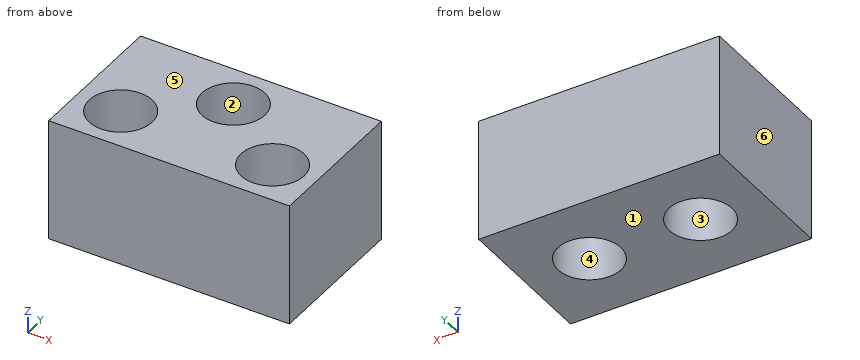
Autodesk Inventor part; units mm, degrees
ref_plane "YZ Plane" through (0, 0, 0) normal (1, 0, 0) x (0, 1, 0)
ref_plane "XZ Plane" through (0, 0, 0) normal (0, 1, 0) x (-1, 0, 0)
ref_plane "XY Plane" through (0, 0, 0) normal (0, 0, 1) x (1, 0, 0)
sketch "Sketch1" plane through (0, 0, 0) normal (0, 0, 1) x (1, 0, 0)
  line L0 (-30.2326, 17.8682) -> (11.0424, 17.8682)
  line L1 (11.0424, 17.8682) -> (11.0424, -7.5318)
  line L2 (11.0424, -7.5318) -> (-30.2326, -7.5318)
  line L3 (-30.2326, -7.5318) -> (-30.2326, 17.8682)
  point P0 (0, 0)
  dimension "d0" = 41.275
  dimension "d1" = 25.4
extrude "Extrusion1" add sketch "Sketch1" along normal blind 20.955
sketch "Sketch2" plane through (0, 0, 20.955) normal (0, 0, 1) x (1, 0, 0)
  line L0 (11.0424, 17.8682) -> (11.0424, -7.5318)
  line L1 (-30.2326, 17.8682) -> (11.0424, 17.8682)
  line L2 (-30.2326, -7.5318) -> (-30.2326, 17.8682)
  line L3 (11.0424, -7.5318) -> (-30.2326, -7.5318)
  circle A0 centre (-9.5951, 10.2482) radius 5.3975
  circle A1 centre (-22.6126, 0.0882) radius 5.3975
  circle A2 centre (3.4224, 0.0882) radius 5.3975
  dimension "d4" = 10.795
  dimension "d5" = 7.62
  dimension "d6" = 7.62
  dimension "d7" = 7.62
  dimension "d8" = 7.62
  dimension "d9" = 7.62
extrude "Extrusion2" cut sketch "Sketch2" against normal blind 9.525 contours A0 | A1 | A2
thread "Thread1"
thread "Thread2"
thread "Thread3"
sketch "Sketch3" plane through (0, 0, 0) normal (0, 0, -1) x (-1, 0, 0)
  line L0 (30.2326, -7.5318) -> (30.2326, 17.8682)
  circle A0 centre (0.0701, 5.1682) radius 5.3975
  circle A1 centre (19.1201, 5.1682) radius 5.3975
  point P0 (0, 0)
  dimension "d18" = 10.795
  dimension "d19" = 19.05
  dimension "d20" = 11.1125
extrude "Extrusion3" cut sketch "Sketch3" against normal blind 9.525
thread "Thread4"
thread "Thread5"
properties part number "Solenoid Base 1764"
Geometry check sheet. Reference: the model listing, model coordinates, mm. Face numbers are marked on the shaded views. A direction names the side the tool comes from. Round coordinates to 2 decimals unless told otherwise and drop trailing zeros. Loops run counter-clockwise (first coordinate to the right, second up) from the corner with the lowest first, then second, coordinate; pieces in that order, holes last. Notation, with made-up numbers: M 52,20.25 L 66,20.25 A27 ccw 66,53.25 Z; hole C -10.75,12 d7. An arc over 180 degrees is marked long. Return JSON: item names as keys, results as strings. Group by question number.
(1) Set-up check for the marked faces 1, 2 and 3: record each of +Z, -Z, +X, -X, +Y, -Y from which the full face is reachable in a straight line by a thin tool's end or side.
(2) Section check D-D, the plane z = 2.75. Enter the section's corners in (x, y) (1 decimal).
(3) Mould release check, pull along X, two halves, no side actions. Record for the marked faces 4, 5 and 6: pulls with the +X half, pulls with the -X half, needs draft (parallel to the pull), parting line crosses it, or undercut.
(4) Section check B-B, the plane y = 15. Enter the section's corners in (x, z) (3 decimals), and give its area (3 significant figures).
(5) Go/stop test with flat-tipped pins: pin 1 (5.5 mm diameter, centred on x = -10.5, y = 9.5, fed in from +Z); pin 2 (8.5 mm diameter, centred on x = -0.07, y = 5.17, fed in from -Z) (3 decimals). Record where each tip stops, or that it passes through.
(6) Section check C-C, the plane x = -9. Enter the section's corners in (y, z) (3 decimals), and give its area (3 significant figures).
(7) Scan lines: line 1 along X through (y, z) = (0.75, 17.5); line 2 along X through (y, z) = (2, 16); line 3 along Z through (x, y) = (-24.5, 2.25). Record each from-to range of solid material in increasing order. Write a range as [from, to].
(8) Section check A-A, the plane z = 15.5. Enter the section's corners in (x, y) (1 decimal).
Data:
{
 "1": {"face 1": "-Z, +X, -X, +Y, -Y", "face 2": "+Z", "face 3": "-Z"},
 "2": {"outline": "M -30.2,-7.5 L 11,-7.5 L 11,17.9 L -30.2,17.9 Z; hole C -19.1,5.2 d10.8; hole C -0.1,5.2 d10.8"},
 "3": {"face 4": "undercut", "face 5": "needs draft", "face 6": "pulls with the -X half"},
 "4": {"outline": "M -30.233,0 L 11.042,0 L 11.042,20.955 L -7.035,20.955 L -7.035,11.43 L -12.155,11.43 L -12.155,20.955 L -30.233,20.955 Z", "area": "816 mm²"},
 "5": {"pin 1": "z = 11.43", "pin 2": "z = 9.525"},
 "6": {"outline": "M -7.532,0 L 17.868,0 L 17.868,20.955 L 15.613,20.955 L 15.613,11.43 L 4.884,11.43 L 4.884,20.955 L -7.532,20.955 Z", "area": "430 mm²"},
 "7": {"line 1": "[-30.23, -27.97], [-17.26, -1.93], [8.78, 11.04]", "line 2": "[-30.23, -27.66], [-17.57, -1.63], [8.47, 11.04]", "line 3": "[0, 11.43]"},
 "8": {"outline": "M -30.2,-7.5 L 11,-7.5 L 11,17.9 L -30.2,17.9 Z; hole C -22.6,0.1 d10.8; hole C -9.6,10.2 d10.8; hole C 3.4,0.1 d10.8"}
}
